Geometry: final body of the model. Coordinates: model frame, mm. A direction names the side the tool comes from. Coordinates: 2 decimals unless noted, no trailing zeros. Order: outer loops, then holes, each group sorted by start corner. A loop starts at its lowest first (then second) coordinate and runs counter-clockwise, first axis right, second up. Notation, with made-up numbers: (50, 39.5) - (88, 39.5) arc R23 ccw to (88, 61.5) - close; hole circle Ø6 at (19, 39). An arc over 180 degrees is marked (long way). Use a Markdown table: item, result. Add a question column.
```python
from build123d import *

# Parameters (mm, degrees)
IZIM1_R                     = 30
Y_KSEKLIK_EKSTR_ZYON1_DEPTH = 20


with BuildPart() as part:
    # Çizim1 → Yükseklik-Ekstrüzyon1 (new body)
    with BuildSketch(Plane.XY):
        with BuildLine():
            Line((-47.124957284, -28.359097323), (-10.82985396, -88.671496349))
            ThreePointArc((-10.82985396, -88.671496349), (-3.536066994, -95.769553672), (6.306494143, -98.359097323))
            Line((6.306494143, -98.359097323), (55, -98.359097323))
            ThreePointArc((55, -98.359097323), (69.142135624, -104.216961699), (75, -118.359097323))
            Line((75, -118.359097323), (75, -148.359097323))
            ThreePointArc((75, -148.359097323), (80.857864376, -162.501232947), (95, -168.359097323))
            Line((95, -168.359097323), (337.882293863, -168.359097323))
            ThreePointArc((337.882293863, -168.359097323), (352.024429487, -162.501232947), (357.882293863, -148.359097323))
            Line((357.882293863, -148.359097323), (357.882293863, -118.359097323))
            ThreePointArc((357.882293863, -118.359097323), (363.740158239, -104.216961699), (377.882293863, -98.359097323))
            Line((377.882293863, -98.359097323), (424.56231333, -98.359097323))
            ThreePointArc((424.56231333, -98.359097323), (435.648622021, -95.005230796), (443.016730749, -86.068473283))
            Line((443.016730749, -86.068473283), (467.124957284, -28.359097323))
            ThreePointArc((467.124957284, -28.359097323), (454.66761994, 42.69843238), (382.566415624, 40.295493058))
            ThreePointArc((382.566415624, 40.295493058), (210, -8.444596477), (37.433584376, 40.295493058))
            ThreePointArc((37.433584376, 40.295493058), (-34.66761994, 42.69843238), (-47.124957284, -28.359097323))
        make_face()
        Circle(IZIM1_R, mode=Mode.SUBTRACT)
        with Locations((420, 0)):
            Circle(IZIM1_R, mode=Mode.SUBTRACT)
    extrude(amount=Y_KSEKLIK_EKSTR_ZYON1_DEPTH)


solid = part.part
```
1) First-contact query: pin 1 (4 mm diameter, centred on y = -35.5, z = 16, fed in from +X); pin 2 (5 mm diameter, centred on y = -111, z = 15, fed in from -X); pin 3 (6 mm diameter, centred on x = 402.5, z = 12.5, fed in from -Y). Flat tips, straight axial feed; report the tip coordinate or a pass-through.
2) Access query for faces 1 (the flat face through (357.882, -134, 10)), 2 (the cylindrical face through (448.615, 9.011, 9.86)), 3 (the flat face through (75, -133, 10)). Directions: +Z, -Z, +X, -X, +Y, -Y. A direction counts if a zero-diameter tool reaches every point of the face in a straight line with its end or side. Return the directions, or none.
3) Section query D-D (x = 87). Return the cut outline in (y, z).
4) Line query: line 1 (Y direction, x = 420, z = 10.5); line 2 (X direction, y = -9.5, z = 9); line 3 (X direction, y = 39.5, z = 12). Output: solid intervals per line, ascending. Write a range as from..to.
5) Section query B-B (y = 0). Return the cut outline in (x, z).
6) Section query C-C (x = 0). Return the cut outline in (y, z), and give its area (3 significant figures).
7) Draft query along Y for faces 4 (the cylindrical face through (435.511, -95.096, 9.86)), 5 (the flat face through (206, -55, 0)), 6 (the cylindrical face through (-29.97, 1.32, 9.86)). Return one class per face: released by +Y, released by -Y, zero draft, split by the parting line, or undercut.
8) Section query A-A (z = 10.5). Return the cut outline in (x, y).
From the geometry:
| question | item | result |
|---|---|---|
| 1 | pin 1 | stops at x = 464.98 |
| 1 | pin 2 | stops at x = 72.4 |
| 1 | pin 3 | stops at y = -98.36 |
| 2 | face 1 | +Z, -Z, +X, -Y |
| 2 | face 2 | +Z, -Z |
| 2 | face 3 | +Z, -Z, -X, -Y |
| 3 | outline | (-166.69, 0) - (15.35, 0) - (15.35, 20) - (-166.69, 20) - close |
| 4 | line 1 | y = -98.36..-30, 30..55 |
| 4 | line 2 | x = -54.17..-28.46, 28.46..391.54, 448.46..474.17 |
| 4 | line 3 | x = -38.27..38.74, 381.26..458.27 |
| 5 | outline | (-55, 0) - (-30, 0) - (-30, 20) - (-55, 20) - close; (30, 0) - (135.84, 0) - (135.84, 20) - (30, 20) - close; (284.16, 0) - (390, 0) - (390, 20) - (284.16, 20) - close; (450, 0) - (475, 0) - (475, 20) - (450, 20) - close |
| 6 | outline | (-97.34, 0) - (-30, 0) - (-30, 20) - (-97.34, 20) - close; (30, 0) - (55, 0) - (55, 20) - (30, 20) - close |
| 6 | area | 1,850 mm^2 |
| 7 | face 4 | released by -Y |
| 7 | face 5 | zero draft |
| 7 | face 6 | undercut |
| 8 | outline | (-47.12, -28.36) - (-10.83, -88.67) arc R20 ccw to (6.31, -98.36) - (55, -98.36) arc R20 cw to (75, -118.36) - (75, -148.36) arc R20 ccw to (95, -168.36) - (337.88, -168.36) arc R20 ccw to (357.88, -148.36) - (357.88, -118.36) arc R20 cw to (377.88, -98.36) - (424.56, -98.36) arc R20 ccw to (443.02, -86.07) - (467.12, -28.36) arc R55 ccw to (382.57, 40.3) arc R329.86 cw to (37.43, 40.3) arc R55 ccw to start; hole circle Ø60 at (0, 0); hole circle Ø60 at (420, 0) |
